Can you work these out from the model? Positions are in its coordinate system, mm. Face numbers are marked on the shaded views. A direction names the side the tool comes from. Coordinates: 2 decimals unless noted, no trailing zeros. Order: outer loops, then holes, each group sorted by start corner. A loop starts at its lowest first (then second) coordinate and runs counter-clockwise, first axis right, second up. Notation, with made-up numbers: (58, -2.75) -> (62, -2.75) arc R16 ccw to (62, 28.25) -> close; hole circle Ø11 at (-34, 9.25). An arc over 180 degrees is marked (long way). Answer as a JSON object with one key per item and string values. Group by question number.
(1) If we mould it in two halves opening along Z, with no side actions, what happens to the marked faces 1, 2 and 3? For each: pulls with the +Z half, pulls with the -Z half, needs draft (parallel to the pull), parting line crosses it, or undercut.
(2) I want a section at B-B, the plane y = -2.8. List the corners of the cut face in (x, z) for me (3 decimals), plus the area to 3 significant figures.
(3) Which directions (+Z, -Z, +X, -X, +Y, -Y) give clear straight access to the entire face, cutting with the end or side of a thin tool? Please do the marked faces 4 and 5.
(4) I want a section at A-A, the plane z = 0. List the corners of the cut face in (x, y) for me (3 decimals), plus the area to 3 significant figures.
(5) I need wall thicknesses on line 1 (X direction, y = -0.65, z = 1.25) (3 decimals); line 2 (Z direction, x = 1, y = -1.5); line 3 (Z direction, x = -10.5, y = -0.55). Which ranges of each line are inside material? Lowest first, please.
(6) I want a section at D-D, the plane z = -2.5. List the corners of the cut face in (x, y) for me (3 decimals).
(7) I want a section at C-C, the plane x = -10. List the corners of the cut face in (y, z) for me (3 decimals).
from build123d import *

# Parameters (mm, degrees)
F0_W     = 31.75
F0_H     = 12.7
F0_R     = 3.175
F0_W_2   = 2.5
F0_H_2   = 6.5
F1_DEPTH = 3.175
F2_R     = 3.175


with BuildPart() as f1:
    # F0 (on Front) → F1 (new body)
    with BuildSketch(Plane.XZ):
        Rectangle(F0_W, F0_H)
        with Locations((-9.525, 0)):
            Circle(F0_R, mode=Mode.SUBTRACT)
        Rectangle(F0_W_2, F0_H_2, mode=Mode.SUBTRACT)
        with Locations((9.525, 0)):
            Rectangle(F0_W_2, F0_H_2, mode=Mode.SUBTRACT)
    extrude(amount=F1_DEPTH)

    # F2
    f2_edges = [f1.edges().sort_by_distance(p)[0] for p in [
        (15.875, -1.5875, -6.35),
        (15.875, -1.5875, 6.35),
        (-15.875, -1.5875, -6.35),
        (-15.875, -1.5875, 6.35),
    ]]
    fillet(f2_edges, radius=F2_R)


solid = f1.part
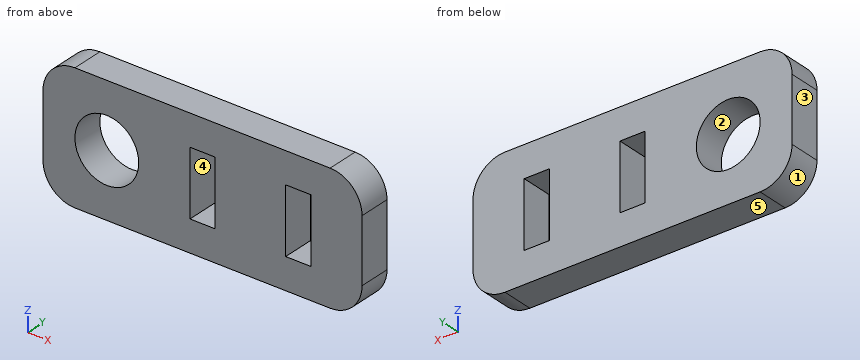
Computed values:
{
 "1": {"face 1": "pulls with the -Z half", "face 2": "undercut", "face 3": "needs draft"},
 "2": {"outline": "(-15.875, -3.175) arc R3.175 ccw to (-12.7, -6.35) -> (12.7, -6.35) arc R3.175 ccw to (15.875, -3.175) -> (15.875, 3.175) arc R3.175 ccw to (12.7, 6.35) -> (-12.7, 6.35) arc R3.175 ccw to (-15.875, 3.175) -> close; hole circle Ø6.35 at (-9.525, 0); hole (-1.25, -3.25) -> (1.25, -3.25) -> (1.25, 3.25) -> (-1.25, 3.25) -> close; hole (8.275, -3.25) -> (10.775, -3.25) -> (10.775, 3.25) -> (8.275, 3.25) -> close", "area": "330 mm2"},
 "3": {"face 4": "+Y, -Y", "face 5": "-Z, +X, -X, +Y, -Y"},
 "4": {"outline": "(-15.875, -3.175) -> (-12.7, -3.175) -> (-12.7, 0) -> (-15.875, 0) -> close; (-6.35, -3.175) -> (-1.25, -3.175) -> (-1.25, 0) -> (-6.35, 0) -> close; (1.25, -3.175) -> (8.275, -3.175) -> (8.275, 0) -> (1.25, 0) -> close; (10.775, -3.175) -> (15.875, -3.175) -> (15.875, 0) -> (10.775, 0) -> close", "area": "64.8 mm2"},
 "5": {"line 1": "x = -15.875 to -12.444, -6.606 to -1.25, 1.25 to 8.275, 10.775 to 15.875", "line 2": "z = -6.35 to -3.25, 3.25 to 6.35", "line 3": "z = -6.35 to -3.02, 3.02 to 6.35"},
 "6": {"outline": "(-15.875, -3.175) -> (-11.482, -3.175) -> (-11.482, 0) -> (-15.875, 0) -> close; (-7.568, -3.175) -> (-1.25, -3.175) -> (-1.25, 0) -> (-7.568, 0) -> close; (1.25, -3.175) -> (8.275, -3.175) -> (8.275, 0) -> (1.25, 0) -> close; (10.775, -3.175) -> (15.875, -3.175) -> (15.875, 0) -> (10.775, 0) -> close"},
 "7": {"outline": "(-3.175, -6.35) -> (0, -6.35) -> (0, -3.139) -> (-3.175, -3.139) -> close; (-3.175, 3.139) -> (0, 3.139) -> (0, 6.35) -> (-3.175, 6.35) -> close"}
}
